from build123d import *

# Parameters (mm, degrees)
F1_DEPTH = 63.5
F2_DEPTH = 25.4
F3_DEPTH = 7.9375


with BuildPart() as f1:
    # F0 (on Front) → F1 (new body, symmetric)
    with BuildSketch(Plane.XZ):
        Polygon((-41.275, 9.525), (-41.275, -9.525), (41.275, -9.525), (41.275, 9.525), (22.225, 9.525), align=None)
    extrude(amount=F1_DEPTH, both=True)

    # F0 (on Front) → F2 (join, symmetric)
    with BuildSketch(Plane.XZ):
        with BuildLine():
            Line((22.225, 9.525), (41.275, 9.525))
            Line((41.275, 9.525), (41.275, 27.076038))
            ThreePointArc((41.275, 27.076038), (45.898045, 38.27466), (57.074575, 42.950859))
            Line((57.074575, 42.950859), (60.325, 42.966303))
            Line((60.325, 42.966303), (60.325, 62.016518))
            Line((60.325, 62.016518), (56.984065, 62.000644))
            add(Edge.make_bspline(
                [(55.727367, 61.972052), (56.147847, 61.983704), (56.566772, 61.993239), (56.984065, 62.000644)],
                knots=[110.259277, 110.259277, 110.259277, 110.259277, 111.393613, 111.393613, 111.393613, 111.393613], degree=3))
            ThreePointArc((55.727367, 61.972052), (31.956339, 51.263537), (22.225, 27.076038))
            Line((22.225, 27.076038), (22.225, 9.525))
        make_face()
        Polygon((85.63449, 62.136769), (60.325, 62.016518), (60.325, 42.966303), (85.725, 43.086984), (85.725, 52.3875), align=None)
    extrude(amount=F2_DEPTH, both=True)

    # F0 (on Front) → F3 (join, symmetric)
    with BuildSketch(Plane.XZ):
        with BuildLine():
            add(Edge.make_bspline(
                [(-41.275, 9.525), (-40.71646, 39.69462), (14.855971, 60.839367), (55.727367, 61.972052)],
                knots=[0, 0, 0, 0, 110.259277, 110.259277, 110.259277, 110.259277], degree=3))
            Line((-41.275, 9.525), (22.225, 9.525))
            Line((22.225, 9.525), (22.225, 27.076038))
            ThreePointArc((22.225, 27.076038), (31.956339, 51.263537), (55.727367, 61.972052))
        make_face()
    extrude(amount=F3_DEPTH, both=True)

    # F0 (on Front) → F4 (revolve)
    with BuildSketch(Plane.XZ):
        Polygon((85.63449, 66.675), (85.63449, 62.136769), (85.725, 52.3875), (85.725, 43.086984), (85.725, 38.1), (111.125, 38.1), (111.125, 66.675), align=None)
    revolve(axis=Axis((85.63449, 0, 64.405885), (0, 0, -1)))


solid = f1.part
Verification items for the finished model (mm, model axes). A direction names the side the tool comes from. Coordinates: 2 decimals unless noted, no trailing zeros. Write each loop counter-clockwise with the first axis right and the second up, starting at its lowest first coordinate (ties: lowest second). Pieces come first, ordered by that corner, then holes. Notation, with made-up numbers: (26.25, 72) - (72.25, 72) arc R24 cw to (72.25, 92) - close; hole circle Ø8 at (32, 48). An arc over 180 degrees is marked (long way). Answer as a JSON object with one key per item and string values.
(1) Cross-section at A-A on x = 66.5. Record the cut outline in (y, z) (3 decimals), plus the area to 3 significant figures.
Report:
{"outline": "(-25.4, 42.996) - (-16.842, 42.996) - (-16.842, 38.1) - (16.842, 38.1) - (16.842, 42.996) - (25.4, 42.996) - (25.4, 62.046) - (16.842, 62.046) - (16.842, 66.675) - (-16.842, 66.675) - (-16.842, 62.046) - (-25.4, 62.046) - close", "area": "1,290 mm^2"}
(2) Cross-section at B-B on y = 46.5. Record the cut outline in (x, z) (3 decimals).
Report:
{"outline": "(-41.275, -9.525) - (41.275, -9.525) - (41.275, 9.525) - (-41.275, 9.525) - close"}
(3) Tool access check on faces 4 (the flat face through (41.275, -1, 4)), 5 (the cylindrical face through (32.217, -16.791, 51.532)), 6 (the flat face through (-3, 7.938, 30)). Record the directions out of +Z, -Z, +X, -X, +Y, -Y that give a thin tool (end or side, any length) a straight path to the whole face; none if there is none.
Report:
{"face 4": "-Z, +X, +Y, -Y", "face 5": "+Z, -X, -Y", "face 6": "+Z, -X, +Y"}
(4) Thickness scan on line 1 along X through (y, z) = (0, 41.15) (3 decimals); line 2 along X through (y, z) = (0, 41.35) (3 decimals); line 3 along X through (y, z) = (51.5, 1.5) (3 decimals). Record the ranges inside material, lowest first.
Report:
{"line 1": "-17.932 to 49.806, 60.144 to 85.544, 85.725 to 111.125", "line 2": "-17.609 to 50.202, 60.144 to 85.544, 85.725 to 111.125", "line 3": "-41.275 to 41.275"}
(5) Gauge pin test, flat ends, axial feed: pin 1 Ø1.5 at (y, z) = (-8.5, 28.5) entering from +X; pin 2 Ø5 at (y, z) = (-22.5, 56) entering from -X; pin 3 Ø15.5 at (x, z) = (11, 30.5) entering from -Y; pin 4 Ø12 at (y, z) = (-36.5, 31) entering from +X. Record the tip position at first contact, or that the pin passes through.
Report:
{"pin 1": "x = 41.42", "pin 2": "x = 34.31", "pin 3": "y = -7.94", "pin 4": "through"}
(6) Mould release check, pull along X, two halves, no side actions. Record for faces 1 (the flat face through (-1, 63.5, 0)), 2 (the flat face through (-41.275, -1, 0)), 3 (the cylindrical face through (45.776, -0.356, 38.151)): pulls with the +X half, pulls with the -X half, needs draft (parallel to the pull), parting line crosses it, or undercut.
Report:
{"face 1": "needs draft", "face 2": "pulls with the -X half", "face 3": "undercut"}
